Read the model definition and answer for the solid it produces. Units are mm, in the model's axes. A direction names the side the tool comes from. Round coordinates to 2 decimals unless told otherwise and drop trailing zeros. Write each loop counter-clockwise with the first axis right and the second up, starting at its lowest first coordinate (ties: lowest second). Pieces come first, ordered by that corner, then holes.
from build123d import *

# Parameters (mm, degrees)
F0_W     = 3
F0_H     = 3
F0_W_2   = 16.1
F0_H_2   = 1.7
F1_DEPTH = 1
F2_DEPTH = 2.5
F3_DEPTH = 2


with BuildPart() as f1:
    # F0 (on Top) → F1 (new body)
    with BuildSketch(Plane.XY):
        with Locations((-11, 10.5)):
            Rectangle(F0_W, F0_H)
        Polygon((9.5, 12), (-9.5, 12), (-9.5, 9), (-12.5, 9), (-12.5, -1), (-9.5, -1), (-9.5, -4), (-12.5, -4), (-12.5, -12), (-8.05, -12), (8.05, -12), (12.5, -12), (12.5, -4), (9.5, -4), (9.5, -1), (12.5, -1), (12.5, 9), (9.5, 9), align=None)
        with Locations((11, 10.5)):
            Rectangle(F0_W, F0_H)
        with Locations((11, -2.5)):
            Rectangle(F0_W, F0_H)
        with Locations((-11, -2.5)):
            Rectangle(F0_W, F0_H)
        with Locations((0, -12.85)):
            Rectangle(F0_W_2, F0_H_2)
    extrude(amount=-F1_DEPTH)

    # F0 (on Top) → F2 (join)
    with BuildSketch(Plane.XY):
        with Locations((-11, 10.5)):
            Rectangle(F0_W, F0_H)
        with Locations((11, 10.5)):
            Rectangle(F0_W, F0_H)
        with Locations((-11, -2.5)):
            Rectangle(F0_W, F0_H)
        with Locations((11, -2.5)):
            Rectangle(F0_W, F0_H)
    extrude(amount=F2_DEPTH)

    # F0 (on Top) → F3 (join)
    with BuildSketch(Plane.XY):
        with Locations((0, -12.85)):
            Rectangle(F0_W_2, F0_H_2)
    extrude(amount=F3_DEPTH)


solid = f1.part
Q1. Determine the mould class of faces 5 (the flat face through (-12.5, -0.2, -0.4)), 6 (the flat face through (0, 0, 0)), 7 (the flat face through (10.2, -12, -0.5)) for opening direction X: pulls with the +X half, pulls with the -X half, needs draft (parallel to the pull), parting line crosses it, or undercut.
Verdict:
face 5: pulls with the -X half
face 6: undercut
face 7: needs draft
Q2. Straight lines are drawn through the part: probe 1 along Y at (x, z) = (10.25, 1.35); probe 2 along Y at (x, z) = (-0.5, 0.35); probe 3 along Z at (x, y) = (5, -5). For each, find the intervals that lie inside material, in ascending order.
Verdict:
probe 1: y = -4 to -1, 9 to 12
probe 2: y = -13.7 to -12
probe 3: z = -1 to 0
Q3. Flat-ended cylindrical pins translate along their axes: pin 1 Ø0.5 at (x, z) = (-11.5, -0.5) entering from -Y; pin 2 Ø0.8 at (x, z) = (-10.5, 1.5) entering from -Y; pin 3 Ø10 at (x, y) = (-3, -0.5) entering from +Z; pin 4 Ø1.9 at (y, z) = (-12.5, 0.5) entering from +X. Find the tip coordinate at first contact, or state that the pin passes through.
Verdict:
pin 1: stops at y = -12
pin 2: stops at y = -4
pin 3: stops at z = 0
pin 4: stops at x = 12.5
Q4. Section A-A (z = 0.95) is taken. Determine the outline of the cut face in (x, y).
Verdict:
outline: (-12.5, -4) - (-9.5, -4) - (-9.5, -1) - (-12.5, -1) - close; (-12.5, 9) - (-9.5, 9) - (-9.5, 12) - (-12.5, 12) - close; (-8.05, -13.7) - (8.05, -13.7) - (8.05, -12) - (-8.05, -12) - close; (9.5, -4) - (12.5, -4) - (12.5, -1) - (9.5, -1) - close; (9.5, 9) - (12.5, 9) - (12.5, 12) - (9.5, 12) - close
Q5. Section C-C (y = -3.25) is taken. Determine the outline of the cut face in (x, z), then the cut area to 3 significant figures.
Verdict:
outline: (-12.5, -1) - (12.5, -1) - (12.5, 2.5) - (9.5, 2.5) - (9.5, 0) - (-9.5, 0) - (-9.5, 2.5) - (-12.5, 2.5) - close
area: 40.0 mm2
Q6. Which of the six approach directions +Z, -Z, +X, -X, +Y, -Y give full straight-line access (tool end or side, diameter ignored) to faces 1 (the flat face through (-11, -1, 1)), 2 (the flat face through (-11, -4, 1)), 3 (the flat face through (0, -12, 1)), 4 (the flat face through (9.5, -3, 1))?
Verdict:
face 1: +Z, +X, -X
face 2: +Z, +X, -X, -Y
face 3: +Z, +X, -X, +Y
face 4: +Z, +Y, -Y
Q7. Section B-B (x = 0) is taken. Determine the outline of the cut face in (y, z), then the cut area to 3 significant figures.
Verdict:
outline: (-13.7, -1) - (12, -1) - (12, 0) - (-12, 0) - (-12, 2) - (-13.7, 2) - close
area: 29.1 mm2
Q8. Section D-D (y = -10.75) is taken. Determine the outline of the cut face in (x, z).
Verdict:
outline: (-12.5, -1) - (12.5, -1) - (12.5, 0) - (-12.5, 0) - close
